CAD build for the part. Positions are in the model's coordinates, mm. Round coordinates to 2 decimals unless told otherwise and drop trailing zeros. Write each loop counter-clockwise with the first axis right and the second up, starting at its lowest first coordinate (ties: lowest second). Pieces come first, ordered by that corner, then holes. Notation, with made-up numbers: (89.25, 4.25) - (145.25, 4.25) arc R17 ccw to (145.25, 12.25) - close; hole circle Ø9 at (28, 37). An arc over 180 degrees is marked (long way). Answer in a Markdown table with one row per item.
```python
from build123d import *

# Parameters (mm, degrees)
ESTRUSIONE_ESTRUSIONE1_DEPTH      = 48
ESTRUSIONE_ESTRUSIONE1_DEPTH_BACK = 5
SCHIZZO2_W                        = 3
SCHIZZO2_H                        = 45
ESTRUSIONE_ESTRUSIONE2_DEPTH      = 5
CORPO_SPOSTA_COPIA1_START         = 29.517316332
CORPO_SPOSTA_COPIA1_OUTLINE_W     = 3
CORPO_SPOSTA_COPIA1_OUTLINE_H     = 43
CORPO_SPOSTA_COPIA1_DEPTH         = 31.678003798
CORPO_SPOSTA_COPIA1_2_OUTLINE_W   = 3
CORPO_SPOSTA_COPIA1_2_OUTLINE_H   = 5
CORPO_SPOSTA_COPIA1_2_DEPTH       = 5
CORPO_SPOSTA_COPIA1_START_2       = 56.19532013
CORPO_SPOSTA_COPIA1_3_OUTLINE_W   = 3
CORPO_SPOSTA_COPIA1_3_OUTLINE_H   = 5
CORPO_SPOSTA_COPIA1_3_DEPTH       = 5
CORPO_SPOSTA_COPIA1_4_OUTLINE_W   = 3
CORPO_SPOSTA_COPIA1_4_OUTLINE_H   = 45
CORPO_SPOSTA_COPIA1_4_DEPTH       = 31.678003798
CORPO_SPOSTA_COPIA1_START_3       = 34.517316332
CORPO_SPOSTA_COPIA1_5_OUTLINE_W   = 3
CORPO_SPOSTA_COPIA1_5_OUTLINE_H   = 3
CORPO_SPOSTA_COPIA1_5_DEPTH       = 21.678003798


# Read off the part's stored shape, not the designer's step: Corpo-Sposta/copia1
with BuildPart() as part:
    # Schizzo1 → Estrusione-Estrusione1 (new, two sides: drawn at the far end of the back side and taken through both)
    with BuildSketch(Plane.XY.offset(-ESTRUSIONE_ESTRUSIONE1_DEPTH_BACK)):
        Polygon((219.519084515, -37.421559693), (210.601374282, -57.180362615), (213.33577775, -58.414476741), (222.253487983, -38.655673819), align=None)
    extrude(amount=ESTRUSIONE_ESTRUSIONE1_DEPTH + ESTRUSIONE_ESTRUSIONE1_DEPTH_BACK)

    # Schizzo2 → Estrusione-Estrusione2 (add)
    with BuildSketch(Plane(origin=(23.117146118, 51.220226082, 0), x_dir=(0.9114678226482943, -0.41137137513052313, 0), z_dir=(0.41137137513052313, 0.9114678226482943, 0))):
        with Locations((216.978740463, -22.5)):
            Rectangle(SCHIZZO2_W, SCHIZZO2_H)
    estrusione_estrusione2 = extrude(amount=ESTRUSIONE_ESTRUSIONE2_DEPTH)

    # Specchia1: Estrusione-Estrusione2 across plane
    add(estrusione_estrusione2.mirror(Plane(origin=(18.658291002, 41.340824621, 0), x_dir=(0, 0, 1), z_dir=(0.41137137513052446, 0.9114678226482937, 0))))

    # Corpo-Sposta/copia1 outline → Corpo-Sposta/copia1 (cut)
    with BuildSketch(Plane(origin=(0, 0, 0), x_dir=(0.9114678226482965, -0.4113713751305183, 0), z_dir=(0.41137137513051825, 0.9114678226482965, 0)).offset(CORPO_SPOSTA_COPIA1_START)):
        with Locations((216.978740463, -26.5)):
            Rectangle(CORPO_SPOSTA_COPIA1_OUTLINE_W, CORPO_SPOSTA_COPIA1_OUTLINE_H)
    extrude(amount=CORPO_SPOSTA_COPIA1_DEPTH, mode=Mode.SUBTRACT)

    # Corpo-Sposta_copia1 2 outline → Corpo-Sposta_copia1 2 (cut)
    with BuildSketch(Plane(origin=(0, 0, 0), x_dir=(0.9114678226482965, -0.4113713751305183, 0), z_dir=(0.41137137513051825, 0.9114678226482965, 0)).offset(CORPO_SPOSTA_COPIA1_START)):
        with Locations((216.978740463, -2.5)):
            Rectangle(CORPO_SPOSTA_COPIA1_2_OUTLINE_W, CORPO_SPOSTA_COPIA1_2_OUTLINE_H)
    extrude(amount=CORPO_SPOSTA_COPIA1_2_DEPTH, mode=Mode.SUBTRACT)

    # Corpo-Sposta_copia1 3 outline → Corpo-Sposta_copia1 3 (cut)
    with BuildSketch(Plane(origin=(0, 0, 0), x_dir=(0.9114678226482965, -0.4113713751305183, 0), z_dir=(0.41137137513051825, 0.9114678226482965, 0)).offset(CORPO_SPOSTA_COPIA1_START_2)):
        with Locations((216.978740463, -2.5)):
            Rectangle(CORPO_SPOSTA_COPIA1_3_OUTLINE_W, CORPO_SPOSTA_COPIA1_3_OUTLINE_H)
    extrude(amount=CORPO_SPOSTA_COPIA1_3_DEPTH, mode=Mode.SUBTRACT)

    # Corpo-Sposta_copia1 4 outline → Corpo-Sposta_copia1 4 (add)
    with BuildSketch(Plane(origin=(0, 0, 0), x_dir=(0.9114678226482965, -0.4113713751305183, 0), z_dir=(0.41137137513051825, 0.9114678226482965, 0)).offset(CORPO_SPOSTA_COPIA1_START)):
        with Locations((216.978740463, 22.5)):
            Rectangle(CORPO_SPOSTA_COPIA1_4_OUTLINE_W, CORPO_SPOSTA_COPIA1_4_OUTLINE_H)
    extrude(amount=CORPO_SPOSTA_COPIA1_4_DEPTH)

    # Corpo-Sposta_copia1 5 outline → Corpo-Sposta_copia1 5 (add)
    with BuildSketch(Plane(origin=(0, 0, 0), x_dir=(0.9114678226482965, -0.4113713751305183, 0), z_dir=(0.41137137513051825, 0.9114678226482965, 0)).offset(CORPO_SPOSTA_COPIA1_START_3)):
        with Locations((216.978740463, 46.5)):
            Rectangle(CORPO_SPOSTA_COPIA1_5_OUTLINE_W, CORPO_SPOSTA_COPIA1_5_OUTLINE_H)
    extrude(amount=CORPO_SPOSTA_COPIA1_5_DEPTH)


solid = part.part
```
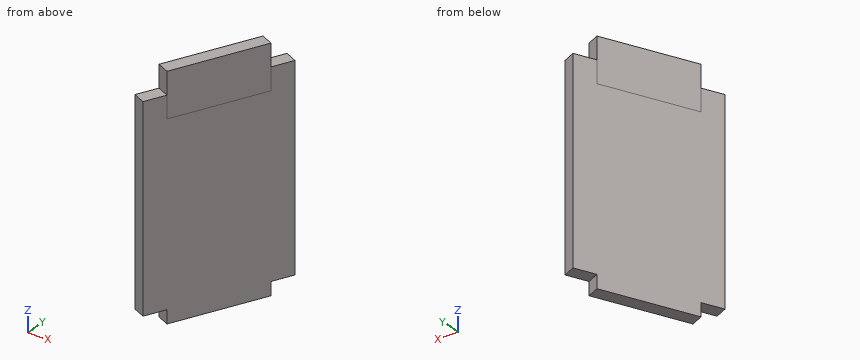
Q1. Saw through at A-A on x = 221. List the corners of the cut face in (y, z).
Computed:
| item | result |
|---|---|
| outline | (-41.43, -48) - (-38.09, -48) - (-38.09, -45) - (-34.14, -45) - (-34.14, 0) - (-38.09, 0) - (-38.09, 5) - (-41.43, 5) - close |
Q2. Saw through at C-C on z = -14. List the corners of the cut face in (x, y), then the cut area to 3 significant figures.
Computed:
| item | result |
|---|---|
| outline | (208.54, -61.74) - (211.28, -62.97) - (224.31, -34.1) - (221.58, -32.86) - close |
| area | 95.0 mm2 |
Q3. Saw through at D-D on x = 212.75. List the corners of the cut face in (y, z), then the cut area to 3 significant figures.
Computed:
| item | result |
|---|---|
| outline | (-59.71, -45) - (-58.15, -45) - (-58.15, -48) - (-52.42, -48) - (-52.42, 5) - (-58.15, 5) - (-58.15, 0) - (-59.71, 0) - close |
| area | 374 mm2 |
Q4. Flat gauge pins, fed straight in: pin 1 (4 mm diameter, centred on x = 210, y = -60.5, fed in from +Z); pin 2 (5.5 mm diameter, centred on x = 222, y = -36.5, fed in from -Z); pin 3 (3 mm diameter, centred on y = -59.5, z = -5, fed in from +X); pin 4 (4 mm diameter, centred on y = -48.5, z = -14, fed in from +X). Where does each tip first touch, or does it go through?
Computed:
| item | result |
|---|---|
| pin 1 | stops at z = 0 |
| pin 2 | stops at z = -48 |
| pin 3 | stops at x = 213.52 |
| pin 4 | stops at x = 218.71 |
Q5. Drill centre lines: line 1 (X direction, y = -59.5, z = -18); line 2 (X direction, y = -51.5, z = -7); line 3 (Y direction, x = 212.5, z = -39). Where is each one in solid material? Low to high.
Computed:
| item | result |
|---|---|
| line 1 | x = 209.55 to 212.85 |
| line 2 | x = 213.17 to 216.46 |
| line 3 | y = -60.27 to -52.97 |
Q6. Saw through at B-B on y = -41. List the corners of the cut face in (x, z).
Computed:
| item | result |
|---|---|
| outline | (217.9, -48) - (221.2, -48) - (221.2, 5) - (217.9, 5) - close |
